```python
from build123d import *

# Parameters (mm, degrees)
F1_DEPTH       = 10
F5_D           = 5
F5_DEPTH       = 8
F5_TIP         = 1.5021515476
F5_ON_F4_D     = 5
F5_ON_F4_DEPTH = 8
F5_ON_F4_TIP   = 1.5021515476
F6_D           = 6.8
F6_DEPTH       = 19
F6_TIP         = 2.0429261047
F8_D           = 4.2
F8_DEPTH       = 10
F8_TIP         = 1.2618073
F10_D          = 5
F10_DEPTH      = 20
F10_TIP        = 1.5021515476
F13_D          = 6.8
F13_DEPTH      = 7
F13_TIP        = 2.0429261047
F14_D          = 5
F14_DEPTH      = 8
F14_TIP        = 1.5021515476
F16_DEPTH      = 5
F17_SIZE       = 1
F18_F1_R       = 1
F18_F2_R       = 1
F18_F3_R       = 1
F18_F4_R       = 1


# Not quite as in the source:
# - a feature names something its author has since deleted; it is built from what else it names


with BuildPart() as f1:
    # F0 (on Front) → F1 (new body, symmetric)
    with BuildSketch(Plane.XZ):
        Polygon((-25.25, 0), (-25.25, -20.4), (-15.25, -20.4), (-15.25, -10), (15.25, -10), (15.25, -20.4), (25.25, -20.4), (25.25, 0), align=None)
    extrude(amount=F1_DEPTH, both=True)

    # F5
    with Locations(Plane(origin=(-25.25, 0, 0), x_dir=(0, -1, 0), z_dir=(-1, 0, 0))):
        with Locations((6, -15.4), (-6, -15.4)):
            Hole(F5_D / 2, depth=F5_DEPTH)
            with Locations((0, 0, -(F5_DEPTH + F5_TIP / 2))):  # 118° drill point
                Cone(0, F5_D / 2, F5_TIP, mode=Mode.SUBTRACT)

    # F5 on F4
    with Locations(Plane.YZ.offset(25.25)):
        with Locations((-6, -15.4), (6, -15.4)):
            Hole(F5_ON_F4_D / 2, depth=F5_ON_F4_DEPTH)
            with Locations((0, 0, -(F5_ON_F4_DEPTH + F5_ON_F4_TIP / 2))):  # 118° drill point
                Cone(0, F5_ON_F4_D / 2, F5_ON_F4_TIP, mode=Mode.SUBTRACT)

    # F6
    with Locations(Plane(origin=(-25.25, 0, 0), x_dir=(0, -1, 0), z_dir=(-1, 0, 0))):
        with Locations((0, -5)):
            Hole(F6_D / 2, depth=F6_DEPTH)
            with Locations((0, 0, -(F6_DEPTH + F6_TIP / 2))):  # 118° drill point
                Cone(0, F6_D / 2, F6_TIP, mode=Mode.SUBTRACT)

    # F8
    with Locations(Plane(origin=(0, 0, -20.4), x_dir=(1, 0, 0), z_dir=(0, 0, -1))):
        with Locations((-20.25, 0), (20.25, 0)):
            Hole(F8_D / 2, depth=F8_DEPTH)
            with Locations((0, 0, -(F8_DEPTH + F8_TIP / 2))):  # 118° drill point
                Cone(0, F8_D / 2, F8_TIP, mode=Mode.SUBTRACT)

    # F10
    with Locations(Plane.XZ.offset(10)):
        with Locations((20.25, -5)):
            Hole(F10_D / 2, depth=F10_DEPTH)
            with Locations((0, 0, -(F10_DEPTH + F10_TIP / 2))):  # 118° drill point
                Cone(0, F10_D / 2, F10_TIP, mode=Mode.SUBTRACT)

    # F13
    with Locations(Plane.XY):
        with Locations((10, 0)):
            Hole(F13_D / 2, depth=F13_DEPTH)
            with Locations((0, 0, -(F13_DEPTH + F13_TIP / 2))):  # 118° drill point
                Cone(0, F13_D / 2, F13_TIP, mode=Mode.SUBTRACT)

    # F14
    with Locations(Plane.XY):
        with Locations((0, 0)):
            Hole(F14_D / 2, depth=F14_DEPTH)
            with Locations((0, 0, -(F14_DEPTH + F14_TIP / 2))):  # 118° drill point
                Cone(0, F14_D / 2, F14_TIP, mode=Mode.SUBTRACT)

    # F15 (on face) → F16 (cut)
    with BuildSketch(Plane.XY):
        with BuildLine():
            Line((-6.75, -6), (-25.25, -6))
            Line((-25.25, -6), (-25.25, -10))
            Line((-25.25, -10), (-3.75, -10))
            ThreePointArc((-3.75, -10), (-4.8106601718, -9.5606601718), (-5.25, -8.5))
            Line((-5.25, -8.5), (-5.25, -7.5))
            ThreePointArc((-5.25, -7.5), (-5.6893398282, -6.4393398282), (-6.75, -6))
        make_face()
        with BuildLine():
            Line((-25.25, 10), (-25.25, 6))
            Line((-25.25, 6), (-6.75, 6))
            ThreePointArc((-6.75, 6), (-5.6893398282, 6.4393398282), (-5.25, 7.5))
            Line((-5.25, 7.5), (-5.25, 8.5))
            ThreePointArc((-5.25, 8.5), (-4.8106601718, 9.5606601718), (-3.75, 10))
            Line((-3.75, 10), (-25.25, 10))
        make_face()
    extrude(amount=-F16_DEPTH, mode=Mode.SUBTRACT)

    # F17
    f17_edges = [f1.edges().sort_by_distance(p)[0] for p in [
        (15.25, 0, -20.4),
        (-15.25, 0, -20.4),
        (-15.25, -10, -15.2),
        (0, -10, -10),
        (15.25, -10, -15.2),
        (0, 10, -10),
        (-15.25, 10, -15.2),
        (15.25, 10, -15.2),
    ]]
    chamfer(f17_edges, length=F17_SIZE)

    # F18: fillet of radius 1 on 16 edges, made by hand

    # F18_f1
    f18_f1_edges = [f1.edges().sort_by_distance(p)[0] for p in [
        (10.75, -10, 0),
        (-4.8106601718, -9.5606601718, 0),
        (-5.25, -8, 0),
        (-5.6893398282, -6.4393398282, 0),
        (-16, -6, 0),
    ]]
    fillet(f18_f1_edges, radius=F18_F1_R)

    # F18_f2
    f18_f2_edges = [f1.edges().sort_by_distance(p)[0] for p in [
        (-16, 6, 0),
        (-5.6893398282, 6.4393398282, 0),
        (-5.25, 8, 0),
        (-4.8106601718, 9.5606601718, 0),
        (10.75, 10, 0),
    ]]
    fillet(f18_f2_edges, radius=F18_F2_R)

    # F18_f3
    f18_f3_edges = [f1.edges().sort_by_distance(p)[0] for p in [
        (-4.8106601718, -9.5606601718, -5),
        (-16, -6, -5),
        (-5.25, -8, -5),
        (-5.6893398282, -6.4393398282, -5),
    ]]
    fillet(f18_f3_edges, radius=F18_F3_R)

    # F18_f4
    f18_f4_edges = [f1.edges().sort_by_distance(p)[0] for p in [
        (-16, 6, -5),
        (-5.6893398282, 6.4393398282, -5),
        (-5.25, 8, -5),
        (-4.8106601718, 9.5606601718, -5),
    ]]
    fillet(f18_f4_edges, radius=F18_F4_R)


solid = f1.part
```
Here's how the part is built. I have some questions about the finished solid (model axes, mm). A direction names the side the tool comes from. Coordinates: 2 decimals unless noted, no trailing zeros. Loops run counter-clockwise (first coordinate to the right, second up) from the corner with the lowest first, then second, coordinate; pieces in that order, holes last. Notation, with made-up numbers: (2, 6.5) - (50, 6.5) arc R7 ccw to (50, 11.5) - close; hole circle Ø2 at (0.25, -14). An arc over 180 degrees is marked (long way). Return JSON: item names as keys, results as strings. Group by question number.
Item 1: If we section it at B-B on x = -9.5: Write out the boundary of the cut face in (y, z).
Item 2: We'd pull the mould along Y, two halves only. Please class faces 1 (the face through (-16.009, 6.094, -15.824)), 2 (the face through (-4.82, 9.55, -2.48)), 3 (the face through (25.25, 0, -10)): +Y half, -Y half, draft (parallel to the pull), parting line (faces both ways), or undercut.
Item 3: If we section it at A-A on z = -12: Write out the boundary of the cut face in (x, y), and give its area (3 significant figures).
Item 4: I need wall thicknesses on line 1 (X direction, y = 8.25, z = -14.25); line 2 (X direction, y = 0, z = -4.25); line 3 (Y direction, x = -21.5, z = -15.4). Which ranges of each line are inside material? Lowest first, please. Write a range as from..to.
Item 5: If we section it at D-D on z = -16.5: State how many separate pieces and enclosed holes the cut face has, and give its area (3 significant figures).
Item 6: Will these pins go through, and if not, where does the flat tip stop? P1, Ø9, axis at x = 10, y = 0, coming from the -Z side; P2, Ø8, axis at x = -14.5, y = 7, coming from the -Z side; P3, Ø1.1, axis at y = 8, z = -2, coming from the -X side; P4, Ø4, axis at y = 6, z = -15.4, coming from the -X side.
Item 7: On a 3-axis mill with a long thin cutter (end or side, diameter ignored), from which of +Z, -Z, +X, -X, +Y, -Y can I reach the whole of each face in a straight line? I mean faces 4 (the face through (15.74, -9.49, -14.62)), 5 (the face through (21.19, 4.66, -13.29)), 6 (the face through (-16, -8, -5)), 7 (the face through (18.247, -0.631, -15.33)), 8 (the face through (-4.949, 8.007, -0.285)). Say none if no direction works.
Item 8: If we section it at C-C on x = 5.5: Write out the boundary of the cut face in (y, z), and give its area (3 significant figures).
Calculated:
{
 "1": {"outline": "(-10, -9) - (-9, -10) - (9, -10) - (10, -9) - (10, -5) - (7, -5) arc R1 cw to (6, -4) - (6, -1) arc R1 ccw to (5, 0) - (-5, 0) arc R1 ccw to (-6, -1) - (-6, -4) arc R1 cw to (-7, -5) - (-10, -5) - close; hole circle Ø6.8 at (0, -5)"},
 "2": {"face 1": "undercut", "face 2": "+Y half", "face 3": "draft"},
 "3": {"outline": "(-25.25, -10) - (-16.25, -10) - (-15.25, -9) - (-15.25, 9) - (-16.25, 10) - (-25.25, 10) - close; (15.25, -9) - (16.25, -10) - (25.25, -10) - (25.25, 10) - (16.25, 10) - (15.25, 9) - close; hole circle Ø4.2 at (-20.25, 0); hole circle Ø4.2 at (20.25, 0)", "area": "370 mm^2"},
 "4": {"line 1": "x = -25.25..-15.25, 15.25..25.25", "line 2": "x = -4.66..-2.5, 2.5..6.6, 13.4..17.87, 22.63..25.25", "line 3": "y = -10..-8.5, -3.5..-1.69, 1.69..3.5, 8.5..10"},
 "5": {"separate pieces": "2", "enclosed holes": "2", "area": "217 mm^2"},
 "6": {"P1": "stops at z = -10", "P2": "stops at z = -20.4", "P3": "stops at x = -5.25", "P4": "stops at x = -16.95"},
 "7": {"face 4": "-Z, -Y", "face 5": "+X", "face 6": "+Z, -X, -Y", "face 7": "-Z", "face 8": "+Z, -X, +Y"},
 "8": {"outline": "(-10, -9) - (-9, -10) - (9, -10) - (10, -9) - (10, -1) arc R1 ccw to (9, 0) - (-9, 0) arc R1 ccw to (-10, -1) - close", "area": "199 mm^2"}
}
